from build123d import *

# Parameters (mm, degrees)
SKETCH1_R           = 2
BOSS_EXTRUDE1_DEPTH = 28
BOSS_EXTRUDE2_DEPTH = 9
SKETCH3_R           = 2
BOSS_EXTRUDE3_DEPTH = 3


with BuildPart() as part:
    # Sketch1 → Boss-Extrude1 (new body)
    with BuildSketch(Plane(origin=(0, 0, 0), x_dir=(1, 0, 0), z_dir=(0, 1, 0))):
        with Locations(Location((0, 0, 0), (0, 0, 270))):
            Circle(SKETCH1_R)
    extrude(amount=BOSS_EXTRUDE1_DEPTH)

    # Sketch2 → Boss-Extrude2 (add)
    with BuildSketch(Plane(origin=(0, 28, 0), x_dir=(1, 0, 0), z_dir=(0, 1, 0))):
        with BuildLine():
            Line((-2, 0), (2, 0))
            ThreePointArc((2, 0), (0, 2), (-2, 0))
        make_face()
    extrude(amount=BOSS_EXTRUDE2_DEPTH)

    # Sketch3 → Boss-Extrude3 (add)
    with BuildSketch(Plane(origin=(0, 37, 0), x_dir=(1, 0, 0), z_dir=(0, 1, 0))):
        with Locations(Location((0, 0, 0), (0, 0, 270))):
            Circle(SKETCH3_R)
    extrude(amount=BOSS_EXTRUDE3_DEPTH)


solid = part.part
Design review of the part built by this model. Coordinates are the model's own, in mm. Coordinates: 2 decimals unless noted, no trailing zeros. Write each loop counter-clockwise with the first axis right and the second up, starting at its lowest first coordinate (ties: lowest second). Pieces come first, ordered by that corner, then holes. Notation, with made-up numbers: (7, 84.25) - (36, 84.25) arc R13 cw to (36, 103.25) - close; hole circle Ø9 at (71, -10). An arc over 180 degrees is marked (long way). Use one line per item in the form item = value.
Q1. For probe 1 along Y at (x, z) = (-0.05, 0.05); probe 2 along Z at (x, y) = (-1.7, 9.5); probe 3 along Z at (x, y) = (-0.85, 31), list the stretches that pass through material, from the lowest coordinate up.
Taken from the geometry:
probe_1 = 0 to 28, 37 to 40
probe_2 = -1.05 to 1.05
probe_3 = -1.81 to 0
Q2. Consider section B-B (z = 0.75). Write out the cut boundary in (x, y).
Taken from the geometry:
outline = (-1.85, 0) - (1.85, 0) - (1.85, 28) - (-1.85, 28) - close; (-1.85, 37) - (1.85, 37) - (1.85, 40) - (-1.85, 40) - close
Q3. Consider section A-A (x = -1.2). Write out the cut boundary in (y, z).
Taken from the geometry:
outline = (0, -1.6) - (40, -1.6) - (40, 1.6) - (37, 1.6) - (37, 0) - (28, 0) - (28, 1.6) - (0, 1.6) - close
Q4. Insertion check: pin 1 Ø1.2 at (x, y) = (0, 33) entering from +Z. The pin has a flat end and moves straight along its axis. Give the tip position at first contact, or say it passes through.
Taken from the geometry:
pin_1 = 0
Q5. The part is to be moulded in two halves that separate along Y. For faces 1 (the cylindrical face through (0, 20, -2)), 2 (the flat face through (0, 40, 0)), 3 (the flat face through (0, 0, 0)), 4 (the flat face through (0, 28, 1)), say which applies: +Y half, -Y half, draft (parallel to the pull), parting line (faces both ways), or undercut.
Taken from the geometry:
face_1 = draft
face_2 = +Y half
face_3 = -Y half
face_4 = undercut
Q6. Consider section D-D (y = 36.5). Write out the cut boundary in (x, z), plus the area to 3 significant figures.
Taken from the geometry:
outline = (-2, 0) arc R2 ccw to (2, 0) - close
area = 6.28 mm^2
Q7. Consider section C-C (y = 20.5). Write out the cut boundary in (x, z).
Taken from the geometry:
outline = circle Ø4 at (0, 0)
